The model under review builds one solid part; all positions refer to its coordinate system, in mm. Coordinates: 2 decimals unless noted, no trailing zeros. Order: outer loops, then holes, each group sorted by start corner. A loop starts at its lowest first (then second) coordinate and runs counter-clockwise, first axis right, second up. Notation, with made-up numbers: M 35,36 L 44,36 A25 cw 44,54 Z; hole C 1,-30 d1. An arc over 180 degrees is marked long. One line per item, written item: value.
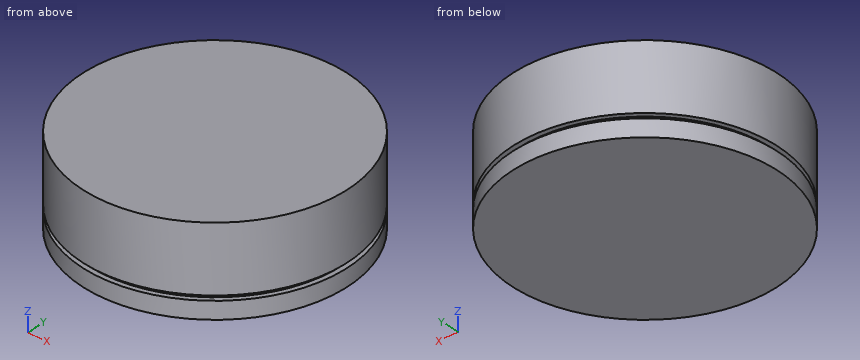
```python
from build123d import *

# Parameters (mm, degrees)
SKETCH1_R           = 38.1
BOSS_EXTRUDE1_DEPTH = 25.4
SKETCH2_W           = 1.476595825
SKETCH2_H           = 1.378223542


with BuildPart() as part:
    # Sketch1 → Boss-Extrude1 (new body)
    with BuildSketch(Plane.XY):
        Circle(SKETCH1_R)
    extrude(amount=BOSS_EXTRUDE1_DEPTH)

    # Sketch2 → Cut-Revolve1 (revolve, cut)
    with BuildSketch(Plane(origin=(0, 0, 0), x_dir=(1, 0, 0), z_dir=(0, 1, 0))):
        with Locations((-37.361702088, -5.660888229)):
            Rectangle(SKETCH2_W, SKETCH2_H)
    revolve(axis=Axis((0, 0, 0), (0, 0, 1)), mode=Mode.SUBTRACT)


solid = part.part
```
(1) We need section C-C, the plane z = 16.25. State the section outline as (x, y) points, plus the area to 3 significant figures.
Geometry results:
outline: C 0,0 d76.2
area: 4,560 mm2
(2) For L1, parallel to Y at x = -3, z = 17.75; L2, parallel to Y at x = -6.5, z = 7.5; L3, parallel to X at y = 9.5, z = 2, list the stretches that pass through material, from the lowest coordinate up.
Geometry results:
L1: y = -37.98 to 37.98
L2: y = -37.54 to 37.54
L3: x = -36.9 to 36.9
(3) We need section B-B, the plane y = -14.5. State the section outline as (x, z) points, plus the area to 3 significant figures.
Geometry results:
outline: M -35.23,0 L 35.23,0 L 35.23,4.97 L 33.63,4.97 L 33.63,6.35 L 35.23,6.35 L 35.23,25.4 L -35.23,25.4 L -35.23,6.35 L -33.63,6.35 L -33.63,4.97 L -35.23,4.97 Z
area: 1,790 mm2
(4) We need section A-A, the plane x = 25.5. State the section outline as (y, z) points.
Geometry results:
outline: M -28.31,0 L 28.31,0 L 28.31,4.97 L 26.29,4.97 L 26.29,6.35 L 28.31,6.35 L 28.31,25.4 L -28.31,25.4 L -28.31,6.35 L -26.29,6.35 L -26.29,4.97 L -28.31,4.97 Z
(5) Insertion check: pin 1 Ø2 at (x, y) = (11.5, 9) entering from -Z; pin 2 Ø6 at (x, z) = (-13.5, 17) entering from +Y; pin 3 Ø2 at (x, z) = (18.5, 15.5) entering from +Y. Each pin has a flat end and moves straight along its axis. Give the tip position at first contact, or say it passes through.
Geometry results:
pin 1: stops at z = 0
pin 2: stops at y = 36.62
pin 3: stops at y = 33.84
